Could you check a few things on this model? Use its own coordinates, in mm. Round coordinates to 2 decimals unless told otherwise and drop trailing zeros. Loops run counter-clockwise (first coordinate to the right, second up) from the corner with the lowest first, then second, coordinate; pieces in that order, holes last. Notation, with made-up numbers: (64, 40.5) -> (74, 40.5) arc R20 ccw to (74, 50.5) -> close; hole circle Ø2 at (75.25, -22.75). An arc over 180 degrees is marked (long way). Write each question's results on one line, items separated by ' | '. Start each with the question number.
1) Imagine slicing it at B-B, the plane z = -2.5. List the corners of the cut face in (x, y) for me.
2) If I drill on probe 1 along X at (y, z) = (1.35, -2.5); probe 2 along X at (y, z) = (1.05, -3.4); probe 3 along Z at (x, y) = (35.5, 1.65), over which ranges is the centre line in solid material (lowest first)?
3) We'd pull the mould along X, two halves only. Please class faces 1 (the cylindrical face through (0, 1, -2.4)), 2 (the flat face through (35, 2, -1)), 3 (the cylindrical face through (1.9, 0.99, -1.76)), 4 (the cylindrical face through (35.99, 1.01, -2.63)): pulls with the +X half, pulls with the -X half, needs draft (parallel to the pull), parting line crosses it, or undercut.
4) Imagine slicing it at C-C, the plane y = 1.6. List the corners of the cut face in (x, z) for me.
5) Imagine slicing it at A-A, the plane x = 35. List the corners of the cut face in (y, z) for me, plus the area to 3 significant figures.
6) For P1, Ø1, axis at y = 0.5, z = -3, coming from the +X side, with a flat end and sliding along its axis, tell me the tip position at first contact or that it passes through.
from build123d import *

# Parameters (mm, degrees)
SKETCH1_W               = 70
SKETCH1_H               = 5
BOSS_EXTRUDE1_DEPTH     = 2
CUT_EXTRUDE1_DEPTH      = 71.206837274
CUT_EXTRUDE1_DEPTH_BACK = 71.206837274
SKETCH2_R               = 1.6
CUT_EXTRUDE2_REACH      = 72.207
SKETCH4_R               = 1
FILLET2_RADIUS          = 2.5
FILLET2_LENGTH          = 2
FILLET3_RADIUS          = 2.5
FILLET3_LENGTH          = 2


with BuildPart() as part:
    # Sketch1 → Boss-Extrude1 (new body)
    with BuildSketch(Plane(origin=(0, 0, 0), x_dir=(1, 0, 0), z_dir=(0, 1, 0))):
        with Locations((35, 2.5)):
            Rectangle(SKETCH1_W, SKETCH1_H)
    extrude(amount=BOSS_EXTRUDE1_DEPTH)

    # Sketch2 → Cut-Extrude1 (cut, two sides: drawn at the far end of the back side and taken through both)
    with BuildSketch(Plane(origin=(0, 2, 0), x_dir=(1, 0, 0), z_dir=(0, 1, 0)).offset(-CUT_EXTRUDE1_DEPTH_BACK)):
        with Locations(Location((66.682907, 2.5, 0), (0, 0, 270))):
            Circle(SKETCH2_R)
        with Locations(Location((3.317093, 2.5, 0), (0, 0, 270))):
            Circle(SKETCH2_R)
    extrude(amount=CUT_EXTRUDE1_DEPTH + CUT_EXTRUDE1_DEPTH_BACK, mode=Mode.SUBTRACT)

    # Sketch4 → Cut-Extrude2 (cut, up to next)
    with BuildSketch(Plane(origin=(0, 2, 0), x_dir=(1, 0, 0), z_dir=(0, 1, 0)), mode=Mode.PRIVATE) as cut_extrude2_sk1:
        with Locations(Location((35, 2.5, 0), (0, 0, 270))):
            Circle(SKETCH4_R)
    cut_extrude2_tool1 = extrude(cut_extrude2_sk1.sketch, amount=-CUT_EXTRUDE2_REACH, mode=Mode.PRIVATE) & part.part
    add(cut_extrude2_tool1.solids().sort_by_distance((35, 2, -2.5))[0], mode=Mode.SUBTRACT)

    # Fillet2: full round fillet: the end face becomes a half cylinder, R = half its width
    fillet2_face = Plane((0, 1, -2.5), x_dir=(0, -1, 0), z_dir=(-1, 0, 0))  # on the end face: x along it, z out of the body
    fillet2_slab = fillet2_face.offset(-FILLET2_RADIUS / 2) * Box(FILLET2_LENGTH, 2 * FILLET2_RADIUS, FILLET2_RADIUS, mode=Mode.PRIVATE)  # the body's end, R deep
    fillet2_round = Plane((2.5, 1, -2.5), x_dir=(-1, 0, 0), z_dir=(0, -1, 0)) * Cylinder(FILLET2_RADIUS, FILLET2_LENGTH, mode=Mode.PRIVATE)  # its axis R under the face
    add(fillet2_slab - fillet2_round, mode=Mode.SUBTRACT)

    # Fillet3: full round fillet: the end face becomes a half cylinder, R = half its width
    fillet3_face = Plane((70, 1, -2.5), x_dir=(0, 1, 0), z_dir=(1, 0, 0))  # on the end face: x along it, z out of the body
    fillet3_slab = fillet3_face.offset(-FILLET3_RADIUS / 2) * Box(FILLET3_LENGTH, 2 * FILLET3_RADIUS, FILLET3_RADIUS, mode=Mode.PRIVATE)  # the body's end, R deep
    fillet3_round = Plane((67.5, 1, -2.5), x_dir=(1, 0, 0), z_dir=(0, 1, 0)) * Cylinder(FILLET3_RADIUS, FILLET3_LENGTH, mode=Mode.PRIVATE)  # its axis R under the face
    add(fillet3_slab - fillet3_round, mode=Mode.SUBTRACT)


solid = part.part
Checked values:
1) outline: (0, 0) -> (1.72, 0) -> (1.72, 2) -> (0, 2) -> close; (4.92, 0) -> (34, 0) -> (34, 2) -> (4.92, 2) -> close; (36, 0) -> (65.08, 0) -> (65.08, 2) -> (36, 2) -> close; (68.28, 0) -> (70, 0) -> (70, 2) -> (68.28, 2) -> close
2) probe 1: 0 to 1.72, 4.92 to 34, 36 to 65.08, 68.28 to 70 | probe 2: 0.17 to 1.99, 4.64 to 34.56, 35.44 to 65.36, 68.01 to 69.83 | probe 3: -5 to -3.37, -1.63 to 0
3) face 1: pulls with the -X half | face 2: needs draft | face 3: undercut | face 4: undercut
4) outline: (2.5, -5) -> (67.5, -5) arc R2.5 ccw to (67.5, 0) -> (2.5, 0) arc R2.5 ccw to start; hole circle Ø3.2 at (3.32, -2.5); hole circle Ø2 at (35, -2.5); hole circle Ø3.2 at (66.68, -2.5)
5) outline: (0, -5) -> (2, -5) -> (2, -3.5) -> (0, -3.5) -> close; (0, -1.5) -> (2, -1.5) -> (2, 0) -> (0, 0) -> close | area: 6.00 mm^2
6) P1: x = 70
